```python
from build123d import *

# Parameters (mm, degrees)
BOSS_EXTRUDE1_DEPTH = 1.8
BOSS_EXTRUDE1_TAPER = 2
SKETCH10_R          = 1.223
CUT_EXTRUDE2_DEPTH  = 0.25
CUT_EXTRUDE2_TAPER  = 2
SKETCH9_R           = 0.815
CUT_EXTRUDE3_DEPTH  = 2.55
CUT_EXTRUDE3_TAPER  = 2
SKETCH12_R          = 0.5
CUT_EXTRUDE4_DEPTH  = 2.8


with BuildPart() as part:
    # Sketch11 → Boss-Extrude1 (new body)
    with BuildSketch(Plane.XY):
        with BuildLine():
            Line((19.812, 0.5), (19.812, 2.683))
            ThreePointArc((19.812, 2.683), (19.519106781, 3.390106781), (18.812, 3.683))
            Line((18.812, 3.683), (-18.812, 3.683))
            ThreePointArc((-18.812, 3.683), (-19.519106781, 3.390106781), (-19.812, 2.683))
            Line((-19.812, 2.683), (-19.812, 0.5))
            Line((-19.812, 0.5), (-19.812, -0.5))
            Line((-19.812, -0.5), (-19.812, -2.683))
            ThreePointArc((-19.812, -2.683), (-19.519106781, -3.390106781), (-18.812, -3.683))
            Line((-18.812, -3.683), (18.812, -3.683))
            ThreePointArc((18.812, -3.683), (19.519106781, -3.390106781), (19.812, -2.683))
            Line((19.812, -2.683), (19.812, -0.5))
            Line((19.812, -0.5), (19.812, 0.5))
        make_face()
    extrude(amount=BOSS_EXTRUDE1_DEPTH, taper=BOSS_EXTRUDE1_TAPER)

    # Sketch10 → Cut-Extrude2 (cut)
    with BuildSketch(Plane.XY):
        with Locations((16.2, 1.885)):
            Circle(SKETCH10_R)
        with Locations((12.6, 1.885)):
            Circle(SKETCH10_R)
        with Locations((9, 1.885)):
            Circle(SKETCH10_R)
        with Locations((5.4, 1.885)):
            Circle(SKETCH10_R)
        with Locations((1.8, 1.885)):
            Circle(SKETCH10_R)
        with Locations((-1.8, 1.885)):
            Circle(SKETCH10_R)
        with Locations((-5.4, 1.885)):
            Circle(SKETCH10_R)
        with Locations((-9, 1.885)):
            Circle(SKETCH10_R)
        with Locations((-12.6, 1.885)):
            Circle(SKETCH10_R)
        with Locations((-16.2, 1.885)):
            Circle(SKETCH10_R)
        with Locations((-18, -1.885)):
            Circle(SKETCH10_R)
        with Locations((-14.4, -1.885)):
            Circle(SKETCH10_R)
        with Locations((-10.8, -1.885)):
            Circle(SKETCH10_R)
        with Locations((-7.2, -1.885)):
            Circle(SKETCH10_R)
        with Locations((-3.6, -1.885)):
            Circle(SKETCH10_R)
        with Locations((0, -1.885)):
            Circle(SKETCH10_R)
        with Locations((3.6, -1.885)):
            Circle(SKETCH10_R)
        with Locations((7.2, -1.885)):
            Circle(SKETCH10_R)
        with Locations((10.8, -1.885)):
            Circle(SKETCH10_R)
        with Locations((14.4, -1.885)):
            Circle(SKETCH10_R)
        with Locations((18, -1.885)):
            Circle(SKETCH10_R)
    extrude(amount=CUT_EXTRUDE2_DEPTH, taper=CUT_EXTRUDE2_TAPER, mode=Mode.SUBTRACT)

    # Sketch9 → Cut-Extrude3 (cut, through all)
    with BuildSketch(Plane.XY.offset(0.25)):
        with Locations((16.2, 1.885)):
            Circle(SKETCH9_R)
        with Locations((12.6, 1.885)):
            Circle(SKETCH9_R)
        with Locations((9, 1.885)):
            Circle(SKETCH9_R)
        with Locations((5.4, 1.885)):
            Circle(SKETCH9_R)
        with Locations((1.8, 1.885)):
            Circle(SKETCH9_R)
        with Locations((-1.8, 1.885)):
            Circle(SKETCH9_R)
        with Locations((-5.4, 1.885)):
            Circle(SKETCH9_R)
        with Locations((-9, 1.885)):
            Circle(SKETCH9_R)
        with Locations((-12.6, 1.885)):
            Circle(SKETCH9_R)
        with Locations((-16.2, 1.885)):
            Circle(SKETCH9_R)
        with Locations((-18, -1.885)):
            Circle(SKETCH9_R)
        with Locations((-14.4, -1.885)):
            Circle(SKETCH9_R)
        with Locations((-10.8, -1.885)):
            Circle(SKETCH9_R)
        with Locations((-7.2, -1.885)):
            Circle(SKETCH9_R)
        with Locations((-3.6, -1.885)):
            Circle(SKETCH9_R)
        with Locations((0, -1.885)):
            Circle(SKETCH9_R)
        with Locations((3.6, -1.885)):
            Circle(SKETCH9_R)
        with Locations((7.2, -1.885)):
            Circle(SKETCH9_R)
        with Locations((10.8, -1.885)):
            Circle(SKETCH9_R)
        with Locations((14.4, -1.885)):
            Circle(SKETCH9_R)
        with Locations((18, -1.885)):
            Circle(SKETCH9_R)
    extrude(amount=CUT_EXTRUDE3_DEPTH, taper=CUT_EXTRUDE3_TAPER, mode=Mode.SUBTRACT)

    # Sketch12 → Cut-Extrude4 (cut, through all)
    with BuildSketch(Plane.XY):
        with Locations((19.812, 0)):
            Circle(SKETCH12_R)
        with Locations((-19.812, 0)):
            Circle(SKETCH12_R)
    extrude(amount=CUT_EXTRUDE4_DEPTH, mode=Mode.SUBTRACT)


solid = part.part
```
The model under review builds one solid part; all positions refer to its coordinate system, in mm. A direction names the side the tool comes from. Round coordinates to 2 decimals unless told otherwise and drop trailing zeros. Order: outer loops, then holes, each group sorted by start corner. A loop starts at its lowest first (then second) coordinate and runs counter-clockwise, first axis right, second up. Notation, with made-up numbers: M -12,70.5 L 35,70.5 A19 cw 35,78.5 Z; hole C -32,-35.5 d1. An arc over 180 degrees is marked long. Use a Markdown table: item, result.
1) Consider section B-B (x = 7.2). Write out the cut boundary in (y, z), then the cut area to 3 significant figures.
Report:
| item | result |
|---|---|
| outline | M -3.68,0 L -3.11,0 L -3.1,0.25 L -2.7,0.25 L -2.65,1.8 L -3.62,1.8 Z; M -1.12,1.8 L -1.07,0.25 L -0.67,0.25 L -0.66,0 L 3.68,0 L 3.62,1.8 Z |
| area | 10.1 mm^2 |
2) Tool access review of faces 1 (the face through (19.312, 0.011, 0.887)), 2 (the face through (14, -1, 0.25)): name each direction out of +Z, -Z, +X, -X, +Y, -Y from which nothing blocks a thin tool from reaching the whole face with its end or side.
Report:
| item | result |
|---|---|
| face 1 | +Z, -Z, +X |
| face 2 | -Z |
3) Consider section A-A (z = 1). Give the number of separate pieces and of enclosed holes in the cut face, then the cut area to 3 significant figures.
Report:
| item | result |
|---|---|
| separate pieces | 1 |
| enclosed holes | 21 |
| area | 246 mm^2 |
4) Wall thickness on line 1 along Z through (x, y) = (-5, 3); line 2 along Y through (x, z) = (-16.5, 1.3); line 3 along Y through (x, z) = (9, 0.85): over which ranges is each line inside the solid? List them lowest first. Write a range as [from, to].
Report:
| item | result |
|---|---|
| line 1 | [0.25, 1.8] |
| line 2 | [-3.64, 1.17], [2.6, 3.64] |
| line 3 | [-3.65, 1.09], [2.68, 3.65] |
5) Insertion check: pin 1 (2.5 mm diameter, centred on x = -7.5, y = -2, fed in from -Z); pin 2 (1.2 mm diameter, centred on x = 7, y = -1.5, fed in from -Z). Each pin has a flat end and moves straight along its axis. Give the tip position at first contact, or say it passes through.
Report:
| item | result |
|---|---|
| pin 1 | z = 0 |
| pin 2 | z = 0.25 |
6) Draft analysis for pull direction Y (two halves, no side actions). For faces 3 (the face through (-14, -1, 0.25)), 4 (the face through (-19.489, 3.375, 0.913)), state which applies: released by +Y, released by -Y, zero draft, split by the parting line, or undercut.
Report:
| item | result |
|---|---|
| face 3 | undercut |
| face 4 | released by +Y |
